```python
from build123d import *

# Parameters (mm, degrees)
SKETCH1_R           = 0.9
BOSS_EXTRUDE1_DEPTH = 5
SKETCH2_R           = 1.6
BOSS_EXTRUDE2_DEPTH = 1.975
SKETCH3_R           = 2.6
BOSS_EXTRUDE3_DEPTH = 1.6


with BuildPart() as part:
    # Sketch1 → Boss-Extrude1 (new, symmetric)
    with BuildSketch(Plane.XY):
        Circle(SKETCH1_R)
    extrude(amount=BOSS_EXTRUDE1_DEPTH, both=True)

    # Sketch2 → Boss-Extrude2 (add, symmetric)
    with BuildSketch(Plane.XY):
        Circle(SKETCH2_R)
    extrude(amount=BOSS_EXTRUDE2_DEPTH, both=True)

    # Sketch3 → Boss-Extrude3 (add)
    with BuildSketch(Plane.XY.offset(5)):
        Circle(SKETCH3_R)
    boss_extrude3 = extrude(amount=BOSS_EXTRUDE3_DEPTH)

    # Mirror1: Boss-Extrude3 across plane
    add(boss_extrude3.mirror(Plane.XY))


solid = part.part
```
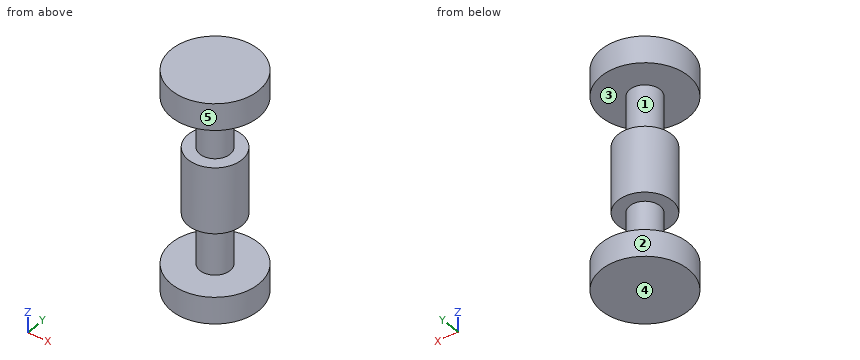
Check sheet for the modelled part. Datum: model origin and axes. Units: mm. Face numbers are marked on the shaded views. A direction names the side the tool comes from. Round coordinates to 2 decimals unless told otherwise and drop trailing zeros. Loops run counter-clockwise (first coordinate to the right, second up) from the corner with the lowest first, then second, coordinate; pieces in that order, holes last. Notation, with made-up numbers: M 10.25,-19 L 29.25,-19 A20 cw 29.25,7 Z; hole C 22,82 d10. An arc over 180 degrees is marked long. Answer as a JSON object with one key per item and string values.
1. Section check D-D (y = -1.4). Record the boundary of the cut face in (x, z) (3 decimals), plus the area to 3 significant figures.
Reply:
{"outline": "M -2.191,-6.6 L 2.191,-6.6 L 2.191,-5 L -2.191,-5 Z; M -2.191,5 L 2.191,5 L 2.191,6.6 L -2.191,6.6 Z; M -0.775,-1.975 L 0.775,-1.975 L 0.775,1.975 L -0.775,1.975 Z", "area": "20.1 mm²"}
2. Gauge pin test, flat ends, axial feed: P1, Ø2, axis at y = -0.5, z = 1, coming from the -X side; P2, Ø2, axis at x = -1.5, z = -2, coming from the -Y side; P3, Ø1.5, axis at x = -1.5, z = -5, coming from the +Y side. Record the tip position at first contact, or that the pin passes through.
Reply:
{"P1": "stops at x = -1.6", "P2": "stops at y = -1.52", "P3": "stops at y = 2.49"}
3. Access from +Z, -Z, +X, -X, +Y, -Y to the whole of each face (thin tool, end or side, straight path). Record for the marked faces 1 and 2.
Reply:
{"face 1": "none", "face 2": "+Z, -Z"}
4. Section check B-B (y = 1.85). Record the boundary of the cut face in (x, z), plus the area to 3 significant figures.
Reply:
{"outline": "M -1.83,-6.6 L 1.83,-6.6 L 1.83,-5 L -1.83,-5 Z; M -1.83,5 L 1.83,5 L 1.83,6.6 L -1.83,6.6 Z", "area": "11.7 mm²"}
5. Scan lines: line 1 (Z direction, x = -1.25, y = -0.6) (3 decimals); line 2 (Z direction, x = 1.7, y = -0.4); line 3 (X direction, y = -0.1, z = 3.25). Record each from-to range of solid material in increasing order.
Reply:
{"line 1": "z = -6.6 to -5, -1.975 to 1.975, 5 to 6.6", "line 2": "z = -6.6 to -5, 5 to 6.6", "line 3": "x = -0.89 to 0.89"}
6. Section check A-A (x = 2.2). Record the boundary of the cut face in (y, z).
Reply:
{"outline": "M -1.39,-6.6 L 1.39,-6.6 L 1.39,-5 L -1.39,-5 Z; M -1.39,5 L 1.39,5 L 1.39,6.6 L -1.39,6.6 Z"}
7. Section check C-C (x = 0). Record the boundary of the cut face in (y, z) (3 decimals).
Reply:
{"outline": "M -2.6,-6.6 L 2.6,-6.6 L 2.6,-5 L 0.9,-5 L 0.9,-1.975 L 1.6,-1.975 L 1.6,1.975 L 0.9,1.975 L 0.9,5 L 2.6,5 L 2.6,6.6 L -2.6,6.6 L -2.6,5 L -0.9,5 L -0.9,1.975 L -1.6,1.975 L -1.6,-1.975 L -0.9,-1.975 L -0.9,-5 L -2.6,-5 Z"}
8. Mould release check, pull along Z, two halves, no side actions. Record for the marked faces 3, 4 and 5: pulls with the +Z half, pulls with the -Z half, needs draft (parallel to the pull), parting line crosses it, or undercut.
Reply:
{"face 3": "undercut", "face 4": "pulls with the -Z half", "face 5": "needs draft"}
